Read the model definition and answer for the solid it produces. Units are mm, in the model's axes. A direction names the side the tool comes from. Round coordinates to 2 decimals unless told otherwise and drop trailing zeros. Loops run counter-clockwise (first coordinate to the right, second up) from the corner with the lowest first, then second, coordinate; pieces in that order, holes last. Notation, with made-up numbers: M 83,21 L 110,21 A22 ccw 110,31 Z; hole C 84.25,57.25 d6. An arc over 180 degrees is marked long. Write each question's results on one line, items separated by ' | '.
```python
from build123d import *

# Parameters (mm, degrees)
CROQUIS1_W              = 220
CROQUIS1_H              = 120
SALIENTE_EXTRUIR1_DEPTH = 5
SALIENTE_EXTRUIR2_DEPTH = 50
CORTAR_EXTRUIR1_REACH   = 173.828
CROQUIS3_R              = 8
CROQUIS3_R_2            = 3.5
CROQUIS3_W              = 12
CROQUIS3_H              = 16
REDONDEO1_R             = 2


with BuildPart() as part:
    # Croquis1 → Saliente-Extruir1 (new body)
    with BuildSketch(Plane(origin=(0, 0, 0), x_dir=(1, 0, 0), z_dir=(0, 1, 0))):
        Rectangle(CROQUIS1_W, CROQUIS1_H)
    extrude(amount=SALIENTE_EXTRUIR1_DEPTH)

    # Croquis2 → Saliente-Extruir2 (add)
    with BuildSketch(Plane(origin=(0, 5, 0), x_dir=(1, 0, 0), z_dir=(0, 1, 0))):
        Polygon((-110, 60), (-105, 60), (105, 60), (110, 60), (110, -60), (105, -60), (105, 55), (-105, 55), (-105, -60), (-110, -60), align=None)
    extrude(amount=SALIENTE_EXTRUIR2_DEPTH)

    # Croquis3 → Cortar-Extruir1 (cut, up to next)
    with BuildSketch(Plane(origin=(0, 0, -60), x_dir=(-1, 0, 0), z_dir=(0, 0, -1)), mode=Mode.PRIVATE) as cortar_extruir1_sk1:
        with Locations((-50, 25)):
            Circle(CROQUIS3_R)
    cortar_extruir1_tool1 = extrude(cortar_extruir1_sk1.sketch, amount=-CORTAR_EXTRUIR1_REACH, mode=Mode.PRIVATE) & part.part
    # Croquis3 → Cortar-Extruir1 (cut, up to next)
    with BuildSketch(Plane(origin=(0, 0, -60), x_dir=(-1, 0, 0), z_dir=(0, 0, -1)), mode=Mode.PRIVATE) as cortar_extruir1_sk2:
        with Locations((10, 25)):
            Circle(CROQUIS3_R)
    cortar_extruir1_tool2 = extrude(cortar_extruir1_sk2.sketch, amount=-CORTAR_EXTRUIR1_REACH, mode=Mode.PRIVATE) & part.part
    # Croquis3 → Cortar-Extruir1 (cut, up to next)
    with BuildSketch(Plane(origin=(0, 0, -60), x_dir=(-1, 0, 0), z_dir=(0, 0, -1)), mode=Mode.PRIVATE) as cortar_extruir1_sk3:
        with Locations((-90, 25)):
            Circle(CROQUIS3_R_2)
    cortar_extruir1_tool3 = extrude(cortar_extruir1_sk3.sketch, amount=-CORTAR_EXTRUIR1_REACH, mode=Mode.PRIVATE) & part.part
    # Croquis3 → Cortar-Extruir1 (cut, up to next)
    with BuildSketch(Plane(origin=(0, 0, -60), x_dir=(-1, 0, 0), z_dir=(0, 0, -1)), mode=Mode.PRIVATE) as cortar_extruir1_sk4:
        with Locations((94, 15)):
            Rectangle(CROQUIS3_W, CROQUIS3_H)
    cortar_extruir1_tool4 = extrude(cortar_extruir1_sk4.sketch, amount=-CORTAR_EXTRUIR1_REACH, mode=Mode.PRIVATE) & part.part
    add(cortar_extruir1_tool1.solids().sort_by_distance((50, 25, -60))[0], mode=Mode.SUBTRACT)
    add(cortar_extruir1_tool2.solids().sort_by_distance((-10, 25, -60))[0], mode=Mode.SUBTRACT)
    add(cortar_extruir1_tool3.solids().sort_by_distance((90, 25, -60))[0], mode=Mode.SUBTRACT)
    add(cortar_extruir1_tool4.solids().sort_by_distance((-94, 15, -60))[0], mode=Mode.SUBTRACT)

    # Redondeo1
    redondeo1_edges = [part.edges().sort_by_distance(p)[0] for p in [
        (-110, 0, 0),
        (0, 0, 60),
        (110, 0, 0),
        (0, 0, -60),
        (-110, 27.5, -60),
        (-110, 27.5, 60),
        (110, 27.5, 60),
        (110, 27.5, -60),
    ]]
    fillet(redondeo1_edges, radius=REDONDEO1_R)


solid = part.part
```
1. Find section A-A, the plane x = 90. Give the vertices of the cut face in (y, z), then the cut area to 3 significant figures.
Completed:
outline: M 0,-58 A2 ccw 2,-60 L 21.5,-60 L 21.5,-55 L 5,-55 L 5,60 L 2,60 A2 ccw 0,58 Z; M 28.5,-60 L 55,-60 L 55,-55 L 28.5,-55 Z | area: 813 mm2
2. Given P1, Ø6, axis at x = -20, z = -26, coming from the +Y side; P2, Ø25, axis at x = 5, y = 22, coming from the +Z side, each flat-ended and moving along its own axis, determine where each tip first touches the part or whether it passes through.
Completed:
P1: stops at y = 5 | P2: stops at z = -55
3. Find section C-C, the plane y = 45. Give the vertices of the cut face in (x, z), then the cut area to 3 significant figures.
Completed:
outline: M -110,-58 A2 ccw -108,-60 L 108,-60 A2 ccw 110,-58 L 110,58 A2 ccw 108,60 L 105,60 L 105,-55 L -105,-55 L -105,60 L -108,60 A2 ccw -110,58 Z | area: 2,250 mm2
4. Which of the six approach directions +Z, -Z, +X, -X, +Y, -Y give full straight-line access (tool end or side, diameter ignored) to faces 1 (the face through (1, 30, -55)), 2 (the face through (-94, 7, -58)), 3 (the face through (1, 3, 60))?
Completed:
face 1: +Z, +Y | face 2: +Z, -Z | face 3: +Z, +X, -X, +Y, -Y
5. Find the intervals of material crossed by L1, parallel to X at y = 8, z = 45; L2, parallel to Z at x = 98, y = 27.5; L3, parallel to Y at x = 50, z = -57.85, in increasing order.
Completed:
L1: x = -110 to -105, 105 to 110 | L2: z = -60 to -55 | L3: y = 0 to 17, 33 to 55
6. Find section B-B, the plane z = 22. Give the vertices of the cut face in (x, y), then the cut area to 3 significant figures.
Completed:
outline: M -110,2 A2 ccw -108,0 L 108,0 A2 ccw 110,2 L 110,55 L 105,55 L 105,5 L -105,5 L -105,55 L -110,55 Z | area: 1,600 mm2
7. Find section D-D, the plane x = -70. Give the vertices of the cut face in (y, z), then the cut area to 3 significant figures.
Completed:
outline: M 0,-58 A2 ccw 2,-60 L 55,-60 L 55,-55 L 5,-55 L 5,60 L 2,60 A2 ccw 0,58 Z | area: 848 mm2
8. Determine the mould class of faces 4 (the face through (86.66, 26.05, -57.54)), 5 (the face through (-1, 5, 2)), 6 (the face through (2, 28, -60)) for opening direction Y: released by +Y, released by -Y, zero draft, split by the parting line, or undercut.
Completed:
face 4: undercut | face 5: released by +Y | face 6: zero draft
